from build123d import *

# Parameters (mm, degrees)
SKETCH1_W           = 68
SKETCH1_H           = 12.192
BOSS_EXTRUDE1_DEPTH = 11.8
SKETCH2_R           = 2.25
CUT_EXTRUDE1_DEPTH  = 13.192
SKETCH3_R           = 4.125
CUT_EXTRUDE2_DEPTH  = 7
SKETCH4_W           = 35
SKETCH4_H           = 12.192
BOSS_EXTRUDE2_DEPTH = 42
SKETCH5_R           = 2.25
CUT_EXTRUDE3_DEPTH  = 13.192
SKETCH6_R           = 4.125
CUT_EXTRUDE4_DEPTH  = 7
CUT_EXTRUDE5_REACH  = 14.192
SKETCH7_R           = 1.25
CHAMFER1_SIZE       = 3.175


with BuildPart() as part:
    # Sketch1 → Boss-Extrude1 (new body)
    with BuildSketch(Plane.XY):
        with Locations((34, -6.096)):
            Rectangle(SKETCH1_W, SKETCH1_H)
    extrude(amount=BOSS_EXTRUDE1_DEPTH)

    # Sketch2 → Cut-Extrude1 (cut, through all)
    with BuildSketch(Plane(origin=(0, 0, 0), x_dir=(1, 0, 0), z_dir=(0, 1, 0))):
        with Locations((39.5, -5.9)):
            Circle(SKETCH2_R)
        with Locations((6, -5.9)):
            Circle(SKETCH2_R)
    extrude(amount=-CUT_EXTRUDE1_DEPTH, mode=Mode.SUBTRACT)

    # Sketch3 → Cut-Extrude2 (cut)
    with BuildSketch(Plane(origin=(0, 0, 0), x_dir=(1, 0, 0), z_dir=(0, 1, 0))):
        with Locations((39.5, -5.9)):
            Circle(SKETCH3_R)
        with Locations((6, -5.9)):
            Circle(SKETCH3_R)
    extrude(amount=-CUT_EXTRUDE2_DEPTH, mode=Mode.SUBTRACT)

    # Sketch4 → Boss-Extrude2 (add)
    with BuildSketch(Plane.XY.offset(11.8)):
        with Locations((17.5, -6.096)):
            Rectangle(SKETCH4_W, SKETCH4_H)
    extrude(amount=BOSS_EXTRUDE2_DEPTH)

    # Sketch5 → Cut-Extrude3 (cut, through all)
    with BuildSketch(Plane(origin=(0, 0, 0), x_dir=(1, 0, 0), z_dir=(0, 1, 0))):
        with Locations((6, -47.8)):
            Circle(SKETCH5_R)
    extrude(amount=-CUT_EXTRUDE3_DEPTH, mode=Mode.SUBTRACT)

    # Sketch6 → Cut-Extrude4 (cut)
    with BuildSketch(Plane(origin=(0, 0, 0), x_dir=(1, 0, 0), z_dir=(0, 1, 0))):
        with Locations((6, -47.8)):
            Circle(SKETCH6_R)
    extrude(amount=-CUT_EXTRUDE4_DEPTH, mode=Mode.SUBTRACT)

    # Sketch7 → Cut-Extrude5 (cut, up to next)
    with BuildSketch(Plane(origin=(0, 0, 0), x_dir=(1, 0, 0), z_dir=(0, 1, 0)), mode=Mode.PRIVATE) as cut_extrude5_sk1:
        with Locations((8.5, -14.400241512)):
            Circle(SKETCH7_R)
    cut_extrude5_tool1 = extrude(cut_extrude5_sk1.sketch, amount=-CUT_EXTRUDE5_REACH, mode=Mode.PRIVATE) & part.part
    add(cut_extrude5_tool1.solids().sort_by_distance((8.5, 0, 14.400242))[0], mode=Mode.SUBTRACT)
    # Sketch7 → Cut-Extrude5 (cut, up to next)
    with BuildSketch(Plane(origin=(0, 0, 0), x_dir=(1, 0, 0), z_dir=(0, 1, 0)), mode=Mode.PRIVATE) as cut_extrude5_sk2:
        with Locations((8.497816512, -37.402425)):
            Circle(SKETCH7_R)
    cut_extrude5_tool2 = extrude(cut_extrude5_sk2.sketch, amount=-CUT_EXTRUDE5_REACH, mode=Mode.PRIVATE) & part.part
    add(cut_extrude5_tool2.solids().sort_by_distance((8.497817, 0, 37.402425))[0], mode=Mode.SUBTRACT)
    # Sketch7 → Cut-Extrude5 (cut, up to next)
    with BuildSketch(Plane(origin=(0, 0, 0), x_dir=(1, 0, 0), z_dir=(0, 1, 0)), mode=Mode.PRIVATE) as cut_extrude5_sk3:
        with Locations((31.5, -37.404608488)):
            Circle(SKETCH7_R)
    cut_extrude5_tool3 = extrude(cut_extrude5_sk3.sketch, amount=-CUT_EXTRUDE5_REACH, mode=Mode.PRIVATE) & part.part
    add(cut_extrude5_tool3.solids().sort_by_distance((31.5, 0, 37.404608))[0], mode=Mode.SUBTRACT)
    # Sketch7 → Cut-Extrude5 (cut, up to next)
    with BuildSketch(Plane(origin=(0, 0, 0), x_dir=(1, 0, 0), z_dir=(0, 1, 0)), mode=Mode.PRIVATE) as cut_extrude5_sk4:
        with Locations((31.502183488, -14.402425)):
            Circle(SKETCH7_R)
    cut_extrude5_tool4 = extrude(cut_extrude5_sk4.sketch, amount=-CUT_EXTRUDE5_REACH, mode=Mode.PRIVATE) & part.part
    add(cut_extrude5_tool4.solids().sort_by_distance((31.502183, 0, 14.402425))[0], mode=Mode.SUBTRACT)

    # Chamfer1
    chamfer1_edges = [part.edges().sort_by_distance(p)[0] for p in [
        (51.5, -12.192, 11.8),
    ]]
    chamfer(chamfer1_edges, length=CHAMFER1_SIZE)


solid = part.part
Geometry: final body of the model. Coordinates: model frame, mm. A direction names the side the tool comes from. Give positions to 0.01 mm unless a question says otherwise; leave off trailing zeros. Write each loop counter-clockwise with the first axis right and the second up, starting at its lowest first coordinate (ties: lowest second). Pieces come first, ordered by that corner, then holes. Notation, with made-up numbers: (73, 15) -> (99, 15) arc R22 ccw to (99, 37) -> close; hole circle Ø3 at (31, -37). An arc over 180 degrees is marked (long way). Answer as a JSON object with one key per item and string values.
1. Cut plane C-C on z = 5.9. Output: boundary loops of the cut face in (x, y) (3 decimals), and give its area (3 significant figures).
Ans:
{"outline": "(0, -12.192) -> (3.75, -12.192) -> (3.75, -7) -> (1.875, -7) -> (1.875, 0) -> (0, 0) -> close; (8.25, -12.192) -> (37.25, -12.192) -> (37.25, -7) -> (35.375, -7) -> (35.375, 0) -> (10.125, 0) -> (10.125, -7) -> (8.25, -7) -> close; (41.75, -12.192) -> (68, -12.192) -> (68, 0) -> (43.625, 0) -> (43.625, -7) -> (41.75, -7) -> close", "area": "667 mm^2"}
2. Ray query, probe 1 along Z at (x, y) = (8.5, -9.5); probe 2 along Z at (x, y) = (6, -1.5) (3 decimals); probe 3 along X at (y, z) = (-10.5, 5.9). Return the intervals inside material, ascending. Write a range as from..to.
Ans:
{"probe 1": "z = 0..13.15, 15.65..36.15, 38.65..53.8", "probe 2": "z = 0..1.775, 10.025..43.675, 51.925..53.8", "probe 3": "x = 0..3.75, 8.25..37.25, 41.75..68"}
3. Mould query, pull axis Z, two halves, no side actions, for faces 5 (the flat face through (17, -6, 53.8)), 6 (the cylindrical face through (8.23, -6.01, 15.62)), 7 (the flat face through (68, -6, 6)). Classes: pulls with the +Z half, pulls with the -Z half, needs draft (parallel to the pull), parting line crosses it, or undercut.
Ans:
{"face 5": "pulls with the +Z half", "face 6": "undercut", "face 7": "needs draft"}
4. Cut plane A-A on z = 47.8. Output: boundary loops of the cut face in (x, y) (3 decimals), and give its area (3 significant figures).
Ans:
{"outline": "(0, -12.192) -> (3.75, -12.192) -> (3.75, -7) -> (1.875, -7) -> (1.875, 0) -> (0, 0) -> close; (8.25, -12.192) -> (35, -12.192) -> (35, 0) -> (10.125, 0) -> (10.125, -7) -> (8.25, -7) -> close", "area": "346 mm^2"}
5. Cut plane D-D on x = 39.5. Output: boundary loops of the cut face in (y, z) (3 decimals), and give its area (3 significant figures).
Ans:
{"outline": "(-12.192, 0) -> (0, 0) -> (0, 1.775) -> (-7, 1.775) -> (-7, 3.65) -> (-12.192, 3.65) -> close; (-12.192, 8.15) -> (-7, 8.15) -> (-7, 10.025) -> (0, 10.025) -> (0, 11.8) -> (-9.017, 11.8) -> (-12.192, 8.625) -> close", "area": "57.7 mm^2"}
6. Cut plane B-B on x = 31.5. Output: boundary loops of the cut face in (y, z).
Ans:
{"outline": "(-12.19, 0) -> (0, 0) -> (0, 13.15) -> (-12.19, 13.15) -> close; (-12.19, 15.65) -> (0, 15.65) -> (0, 36.15) -> (-12.19, 36.15) -> close; (-12.19, 38.65) -> (0, 38.65) -> (0, 53.8) -> (-12.19, 53.8) -> close"}
7. Access query for faces 1 (the flat face through (34, -6, 0)), 2 (the flat face through (51, -4, 11.8)), 3 (the flat face through (8, -7, 8)), 4 (the flat face through (51.269, -10.582, 10.235)). Directions: +Z, -Z, +X, -X, +Y, -Y. A direction counts if a zero-diameter tool reaches every point of the face in a straight line with its end or side. Return the directions, or none.
Ans:
{"face 1": "-Z, +X, -X, +Y, -Y", "face 2": "+Z, +X, +Y, -Y", "face 3": "+Y", "face 4": "+Z, +X, -Y"}
8. Contact query for flat-ended pins moving along their axis: pin 1 (2 mm diameter, centred on x = 8.5, z = 14.4, fed in from -Y); pin 2 (5 mm diameter, centred on x = 39.5, z = 5.9, fed in from +Y); pin 3 (2.5 mm diameter, centred on x = 55.5, y = -6.5, fed in from +Z). Output: stop coordinate, or through.
Ans:
{"pin 1": "passes through", "pin 2": "stops at y = -7", "pin 3": "stops at z = 11.8"}
